Input: part model. Units: mm. Frame: model coordinates. A direction names the side the tool comes from. Round coordinates to 2 decimals unless told otherwise and drop trailing zeros. Loops run counter-clockwise (first coordinate to the right, second up) from the corner with the lowest first, then second, coordinate; pieces in that order, holes last. Notation, with made-up numbers: (-27, -23.75) -> (-4, -23.75) arc R13 cw to (-4, -7.75) -> close; hole circle Ø2 at (-9.75, 74.5). An arc over 180 degrees is marked (long way). Answer in a Markdown table with one row per item. Add a question column.
Q1. Section A-A, the plane y = 9. Output: boundary loops of the cut face in (x, z), and give its area (3 significant figures).
Q2. Section B-B, the plane y = -18.5. Output: boundary loops of the cut face in (x, z), and give its area (3 significant figures).
Q3. Pin query (flat end, axial travel): pin 1 (1 mm diameter, centred on y = -10.5, z = 0, fed in from +X); pin 2 (6 mm diameter, centred on x = 7, y = -11, fed in from +Z); pin 3 (5 mm diameter, centred on x = -8.5, z = 4, fed in from -Y). Return the tip coordinate at first contact, or that it passes through.
Q4. Mould query, pull axis Z, two halves, no side actions, for faces 3 (the face through (-5, 0, 5)), 4 (the face through (-2.435, -12.862, 0.767)), 5 (the face through (-5.13, -12.47, 2.67)). Classes: pulls with the +Z half, pulls with the -Z half, needs draft (parallel to the pull), parting line crosses it, or undercut.
Q5. Reachability of faces 1 (the face through (1.24, -24.13, -2.41)), 2 (the face through (0, 3.175, 0)) from +Z, -Z, +X, -X, +Y, -Y: full face, straight path, thin tool, end or side. Return the list, or none.
Q6. Ray query, L1, parallel to Y at x = -8.5, z = 8; L2, parallel to Z at x = 0, y = -17; L3, parallel to Y at x = 3.5, z = 7 (3 decimals). Return the intervals inside material, ascending. Write a range as from..to.
```python
from build123d import *

# Parameters (mm, degrees)
F3_D     = 5.1054
F3_DEPTH = 22.225
F3_TIP   = 1.5338169022
F4_R     = 0.762
F5_R     = 0.254


with BuildPart() as f1:
    # F0 (on Right) → F1 (revolve)
    with BuildSketch(Plane.YZ):
        Polygon((-24.13, 0), (25.4, 0), (25.4, 12.7), (0, 12.7), (0, 6.096), (-24.13, 5.4941811878), align=None)
    revolve(axis=Axis((0, 0.635, 0), (0, 1, 0)))

    # F3
    with Locations(Plane.XZ.offset(24.13)):
        with Locations((0, 0)):
            Hole(F3_D / 2, depth=F3_DEPTH)
            with Locations((0, 0, -(F3_DEPTH + F3_TIP / 2))):  # 118° drill point
                Cone(0, F3_D / 2, F3_TIP, mode=Mode.SUBTRACT)

    # F4
    f4_edges = [f1.edges().sort_by_distance(p)[0] for p in [
        (0, 0, -6.096),
    ]]
    fillet(f4_edges, radius=F4_R)

    # F5
    f5_edges = [f1.edges().sort_by_distance(p)[0] for p in [
        (0, 0, -12.7),
        (0, -24.13, -5.494181),
    ]]
    fillet(f5_edges, radius=F5_R)

    # F6 (on Right) → F7 (revolve, cut)
    with BuildSketch(Plane.YZ):
        Polygon((3.175, 0), (25.4, 0), (25.4, 8.7376), (3.175, 7.961485898), align=None)
    revolve(axis=Axis((0, 14.2875, 0), (0, -1, 0)), mode=Mode.SUBTRACT)


solid = f1.part
```
Answer block:
| question | item | result |
|---|---|---|
| 1 | outline | circle Ø25.4 at (0, 0); hole circle Ø16.33 at (0, 0) |
| 1 | area | 297 mm^2 |
| 2 | outline | circle Ø11.27 at (0, 0); hole circle Ø5.11 at (0, 0) |
| 2 | area | 79.3 mm^2 |
| 3 | pin 1 | x = 5.85 |
| 3 | pin 2 | z = 4.23 |
| 3 | pin 3 | y = 0 |
| 4 | face 3 | needs draft |
| 4 | face 4 | undercut |
| 4 | face 5 | parting line crosses it |
| 5 | face 1 | +Z, -Z, +X, -X, -Y |
| 5 | face 2 | +Y |
| 6 | L1 | 0..25.4 |
| 6 | L2 | -5.67..-2.55, 2.55..5.67 |
| 6 | L3 | 0..3.175 |
